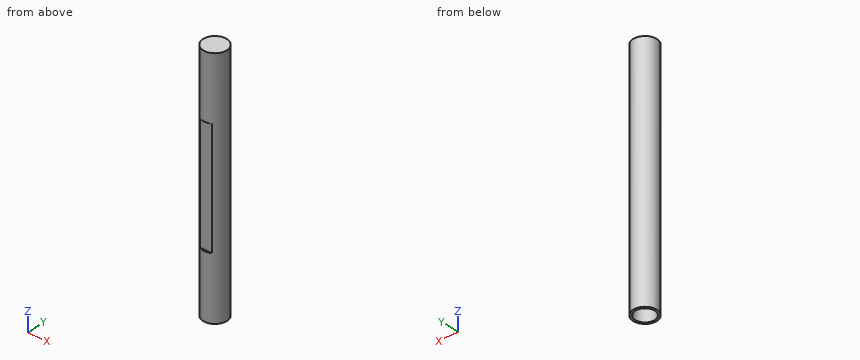
```python
from build123d import *

# Parameters (mm, degrees)
SKETCH1_R           = 5.6
SKETCH1_R_2         = 4.6
BOSS_EXTRUDE1_DEPTH = 115
SKETCH1_3_R         = 4.6
CUT_EXTRUDE1_DEPTH  = 113
SKETCH2_W           = 5.5
SKETCH2_H           = 1.489117796
CUT_EXTRUDE2_DEPTH  = 55


with BuildPart() as part:
    # Sketch1 → Boss-Extrude1 (new body)
    # profile 1 of 2: a face of its own
    with BuildSketch(Plane.XY):
        Circle(SKETCH1_R)
        Circle(SKETCH1_R_2, mode=Mode.SUBTRACT)
    # profile 2 of 2: a face of its own
    with BuildSketch(Plane.XY):
        Circle(SKETCH1_R_2)
    extrude(amount=BOSS_EXTRUDE1_DEPTH)

    # Sketch1_3 → Cut-Extrude1 (cut)
    with BuildSketch(Plane.XY):
        Circle(SKETCH1_3_R)
    extrude(amount=CUT_EXTRUDE1_DEPTH, mode=Mode.SUBTRACT)

    # Sketch2 → Cut-Extrude2 (cut)
    with BuildSketch(Plane.XY.offset(85)):
        with Locations((0, -5.6)):
            Rectangle(SKETCH2_W, SKETCH2_H)
    extrude(amount=-CUT_EXTRUDE2_DEPTH, mode=Mode.SUBTRACT)


solid = part.part
```
Source: CAD feature listing. Evaluate the final solid. Frame: model axes, mm. Coordinates: 2 decimals unless noted, no trailing zeros. Write each loop counter-clockwise with the first axis right and the second up, starting at its lowest first coordinate (ties: lowest second). Pieces come first, ordered by that corner, then holes. Notation, with made-up numbers: (82, 57.25) -> (93, 57.25) arc R30 ccw to (93, 93.25) -> close; hole circle Ø3 at (84.5, -1). An arc over 180 degrees is marked (long way). Return JSON: item names as keys, results as strings. Group by question number.
1) Contact query for flat-ended pins moving along their axis: P1, Ø1, axis at y = 3.5, z = 87.5, coming from the +X side; P2, Ø3, axis at x = -0.5, z = 50.5, coming from the -Y side; P3, Ø3, axis at x = -1, y = 1, coming from the -Z side. Output: stop coordinate, or through.
2) Section query A-A, the plane x = 0. Return loops of the section in (y, z), plus the area to 3 significant figures.
3) Section query B-B, the plane y = 0. Return loops of the section in (x, z).
4) Ray query, line 1 along Y through (x, z) = (0, 49); line 2 along Z through (x, y) = (0.75, 2); line 3 along X through (y, z) = (-3.5, 20). Return the intervals inside material, ascending.
5) Section query C-C, the plane z = 104.5. Return loops of the section in (x, y).
From the geometry:
{
 "1": {"P1": "x = 4.73", "P2": "y = -4.86", "P3": "z = 113"},
 "2": {"outline": "(-5.6, 0) -> (-4.6, 0) -> (-4.6, 113) -> (4.6, 113) -> (4.6, 0) -> (5.6, 0) -> (5.6, 115) -> (-5.6, 115) -> (-5.6, 85) -> (-4.86, 85) -> (-4.86, 30) -> (-5.6, 30) -> close", "area": "207 mm²"},
 "3": {"outline": "(-5.6, 0) -> (-4.6, 0) -> (-4.6, 113) -> (4.6, 113) -> (4.6, 0) -> (5.6, 0) -> (5.6, 115) -> (-5.6, 115) -> close"},
 "4": {"line 1": "-4.86 to -4.6, 4.6 to 5.6", "line 2": "113 to 115", "line 3": "-4.37 to -2.98, 2.98 to 4.37"},
 "5": {"outline": "circle Ø11.2 at (0, 0); hole circle Ø9.2 at (0, 0)"}
}
